from build123d import *

# Parameters (mm, degrees)
SKETCH1_R           = 33
BOSS_EXTRUDE1_DEPTH = 4
BOSS_EXTRUDE2_DEPTH = 3
SKETCH3_R           = 4
BOSS_EXTRUDE3_DEPTH = 78
SKETCH4_R           = 4
BOSS_EXTRUDE4_DEPTH = 150


with BuildPart() as part:
    # Sketch1 → Boss-Extrude1 (new body)
    with BuildSketch(Plane(origin=(0, 0, 0), x_dir=(1, 0, 0), z_dir=(0, 1, 0))):
        with Locations(Location((0, 0, 0), (0, 0, 270))):
            Circle(SKETCH1_R)
    extrude(amount=BOSS_EXTRUDE1_DEPTH)

    # Sketch2 → Boss-Extrude2 (add)
    with BuildSketch(Plane(origin=(0, 4, 0), x_dir=(1, 0, 0), z_dir=(0, 1, 0))):
        with BuildLine():
            ThreePointArc((18, 0), (30.727922061, 30.727922061), (0, 18))
            ThreePointArc((0, 18), (-30.727922061, 30.727922061), (-18, 0))
            ThreePointArc((-18, 0), (-30.727922061, -30.727922061), (0, -18))
            ThreePointArc((0, -18), (30.727922061, -30.727922061), (18, 0))
        make_face()
    extrude(amount=BOSS_EXTRUDE2_DEPTH)

    # Sketch3 → Boss-Extrude3 (add)
    with BuildSketch(Plane(origin=(0, 7, 0), x_dir=(1, 0, 0), z_dir=(0, 1, 0))):
        with Locations(Location((-18, 18, 0), (0, 0, 270))):
            Circle(SKETCH3_R)
        with Locations(Location((18, 18, 0), (0, 0, 270))):
            Circle(SKETCH3_R)
        with Locations(Location((18, -18, 0), (0, 0, 270))):
            Circle(SKETCH3_R)
        with Locations(Location((-18, -18, 0), (0, 0, 270))):
            Circle(SKETCH3_R)
    extrude(amount=BOSS_EXTRUDE3_DEPTH)

    # Sketch4 → Boss-Extrude4 (add)
    with BuildSketch(Plane(origin=(0, 7, 0), x_dir=(1, 0, 0), z_dir=(0, 1, 0))):
        with Locations(Location((0, 0, 0), (0, 0, 270))):
            Circle(SKETCH4_R)
    extrude(amount=BOSS_EXTRUDE4_DEPTH)


solid = part.part
The listing builds one solid part. Answer for the finished solid, in the listing's coordinates (mm). A direction names the side the tool comes from. Coordinates: 2 decimals unless noted, no trailing zeros. Write each loop counter-clockwise with the first axis right and the second up, starting at its lowest first coordinate (ties: lowest second). Pieces come first, ordered by that corner, then holes. Notation, with made-up numbers: (51.5, 27.5) -> (99.5, 27.5) arc R12 ccw to (99.5, 41.5) -> close; hole circle Ø1 at (-25.5, -24.5). An arc over 180 degrees is marked (long way). One line per question, with ' | ' between items.
1. Section B-B (x = 30.5) is taken. Determine the outline of the cut face in (y, z), and give its area (3 significant figures).
Verdict:
outline: (0, -12.6) -> (4, -12.6) -> (4, -30.95) -> (7, -30.95) -> (7, -5.05) -> (4, -5.05) -> (4, 5.05) -> (7, 5.05) -> (7, 30.95) -> (4, 30.95) -> (4, 12.6) -> (0, 12.6) -> close | area: 256 mm^2
2. Which of the six approach directions +Z, -Z, +X, -X, +Y, -Y give full straight-line access (tool end or side, diameter ignored) to faces 4 (the flat face through (0, 4, -29)), 5 (the flat face through (-25, 4, 25)), 6 (the flat face through (-1, 7, -9)), 7 (the flat face through (-25, 4, -25)), 8 (the flat face through (-18, 85, 18))?
Verdict:
face 4: -Z, +Y | face 5: +Z, -X, -Y | face 6: +Y | face 7: -Z, -X, -Y | face 8: +Z, -Z, +X, -X, +Y
3. Given pin 1 Ø1 at (x, y) = (-1.5, 64) entering from +Z; pin 2 Ø2 at (x, z) = (23.5, -26.5) entering from -Y; pin 3 Ø10 at (x, y) = (4, 34) entering from +Z, each flat-ended and moving along its own axis, determine where each tip first touches the part or whether it passes through.
Verdict:
pin 1: stops at z = 3.87 | pin 2: stops at y = 4 | pin 3: stops at z = 4
4. Straight lines are drawn through the part: line 1 (Z direction, x = 17.5, y = 78); line 2 (Y direction, x = -21.5, z = -28.5). For each, find the intervals that lie inside material, in ascending order.
Verdict:
line 1: z = -21.97 to -14.03, 14.03 to 21.97 | line 2: y = 4 to 7
5. Section D-D (y = 144) is taken. Determine the outline of the cut face in (x, z), and give its area (3 significant figures).
Verdict:
outline: circle Ø8 at (0, 0) | area: 50.3 mm^2
6. Section C-C (z = 2) is taken. Determine the outline of the cut face in (x, y).
Verdict:
outline: (-32.94, 0) -> (32.94, 0) -> (32.94, 4) -> (26.25, 4) -> (26.25, 7) -> (3.46, 7) -> (3.46, 157) -> (-3.46, 157) -> (-3.46, 7) -> (-26.25, 7) -> (-26.25, 4) -> (-32.94, 4) -> close
7. Section A-A (y = 78.5) is taken. Determine the outline of the cut face in (x, z), and give its area (3 significant figures).
Verdict:
outline: circle Ø8 at (-18, -18); circle Ø8 at (-18, 18); circle Ø8 at (0, 0); circle Ø8 at (18, -18); circle Ø8 at (18, 18) | area: 251 mm^2
8. For a pull along Z with two mould halves and no side action, classify faces 1 (the flat face through (0, 4, 29)), 2 (the cylindrical face through (-32.215, 1.972, -7.154)), 3 (the cylindrical face through (-31.14, 5.48, 30.3)) as released by +Z, released by -Z, zero draft, split by the parting line, or undercut.
Verdict:
face 1: zero draft | face 2: split by the parting line | face 3: undercut
